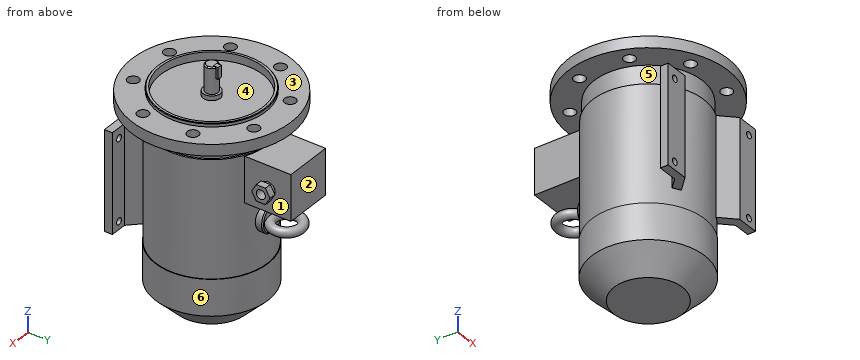
```python
from build123d import *

# Parameters (mm, degrees)
SKETCH_1_R           = 5.5
EXTRUDE_1_DEPTH      = 23
SKETCH_2_W           = 4
SKETCH_2_H           = 4
EXTRUDE_2_DEPTH      = 0.1
EXTRUDE_2_DEPTH_BACK = 10
SKETCH_3_R           = 7.5
EXTRUDE_11_DEPTH     = 4
SKETCH_16_R          = 70
SKETCH_16_R_2        = 47.5
EXTRUDE_13_DEPTH     = 10
SKETCH_17_R          = 47.5
EXTRUDE_14_DEPTH     = 23
SKETCH_18_R          = 5
CUT_EXTRUDE_4_DEPTH  = 28
SKETCH_20_R          = 49
EXTRUDE_15_DEPTH     = 102
SKETCH_21_R          = 49.5
EXTRUDE_16_DEPTH     = 51
CHAMFER_3_SIZE       = 19.5
EXTRUDE_17_DEPTH     = 87
CUT_EXTRUDE_5_REACH  = 128
SKETCH_23_R          = 2.9
SKETCH_24_W          = 42
SKETCH_24_H          = 40
EXTRUDE_18_DEPTH     = 43
SKETCH_25_R          = 12.5
EXTRUDE_19_DEPTH     = 12
CHAMFER_4_SIZE       = 1
SKETCH_27_R          = 4
CHAMFER_5_SIZE       = 1
SKETCH_28_R          = 47.5
SKETCH_28_R_2        = 45
EXTRUDE_20_DEPTH     = 7
CHAMFER_6_SIZE       = 0.5
SKETCH_29_R          = 6
EXTRUDE_21_DEPTH     = 3
EXTRUDE_22_DEPTH     = 6
SKETCH_31_R          = 4
CUT_EXTRUDE_6_DEPTH  = 10


with BuildPart() as part:
    # Sketch 1 → Extrude 1 (new body)
    with BuildSketch(Plane.XY):
        Circle(SKETCH_1_R)
    extrude(amount=EXTRUDE_1_DEPTH)

    # Sketch 2 → Extrude 2 (add, two sides)
    with BuildSketch(Plane.XY.offset(23)) as extrude_2_sk:
        with Locations((0, 5)):
            Rectangle(SKETCH_2_W, SKETCH_2_H)
    extrude(amount=EXTRUDE_2_DEPTH)
    extrude(extrude_2_sk.sketch, amount=-EXTRUDE_2_DEPTH_BACK)

    # Sketch 3 → Extrude 11 (add)
    with BuildSketch(Plane(origin=(0, 0, 0), x_dir=(-1, 0, 0), z_dir=(0, 0, -1))):
        Circle(SKETCH_3_R)
    extrude(amount=EXTRUDE_11_DEPTH)



with BuildPart() as body_2:
    # Sketch 16 → Extrude 13 (new body)
    with BuildSketch(Plane.XY):
        Circle(SKETCH_16_R)
        Circle(SKETCH_16_R_2, mode=Mode.SUBTRACT)
    extrude(amount=-EXTRUDE_13_DEPTH)


with BuildPart() as part_1:
    add(part.part)

    add(body_2.part)  # Extrude 14 merges body 2
    # Sketch 17 → Extrude 14 (add)
    with BuildSketch(Plane(origin=(0, 0, -4), x_dir=(-1, 0, 0), z_dir=(0, 0, -1))):
        with Locations(Location((0, 0, 0), (0, 0, 180))):  # turned: the seam where the file's is
            Circle(SKETCH_17_R)
    extrude(amount=EXTRUDE_14_DEPTH)

    # Sketch 18 → Cut-Extrude 4 (cut, through all)
    with BuildSketch(Plane.XY):
        with Locations((-22.004297361, 53.123073119)):
            Circle(SKETCH_18_R)
        with Locations((22.004297361, 53.123073119)):
            Circle(SKETCH_18_R)
        with Locations((53.123073119, 22.004297361)):
            Circle(SKETCH_18_R)
        with Locations((53.123073119, -22.004297361)):
            Circle(SKETCH_18_R)
        with Locations((22.004297361, -53.123073119)):
            Circle(SKETCH_18_R)
        with Locations((-22.004297361, -53.123073119)):
            Circle(SKETCH_18_R)
        with Locations((-53.123073119, -22.004297361)):
            Circle(SKETCH_18_R)
        with Locations((-53.123073119, 22.004297361)):
            Circle(SKETCH_18_R)
    extrude(amount=-CUT_EXTRUDE_4_DEPTH, mode=Mode.SUBTRACT)

    # Sketch 20 → Extrude 15 (add)
    with BuildSketch(Plane(origin=(0, 0, -27), x_dir=(-1, 0, 0), z_dir=(0, 0, -1))):
        Circle(SKETCH_20_R)
    extrude(amount=EXTRUDE_15_DEPTH)

    # Sketch 21 → Extrude 16 (add)
    with BuildSketch(Plane(origin=(0, 0, -129), x_dir=(-1, 0, 0), z_dir=(0, 0, -1))):
        Circle(SKETCH_21_R)
    extrude(amount=EXTRUDE_16_DEPTH)

    # Chamfer 3
    chamfer_3_edges = [part_1.edges().sort_by_distance(p)[0] for p in [
        (49.5, 0, -180),
    ]]
    chamfer(chamfer_3_edges, length=CHAMFER_3_SIZE)

    # Sketch 22 → Extrude 17 (add)
    with BuildSketch(Plane.XY.offset(-27)):
        with BuildLine():
            Line((-53, -49), (-53, -56))
            Line((-53, -56), (-44.904134404, -56))
            Line((-44.904134404, -56), (-42, -56))
            Line((-42, -56), (-32.646287703, -56))
            Line((-32.646287703, -56), (-20.944471698, -44.298183995))
            ThreePointArc((-20.944471698, -44.298183995), (-24.169591816, -42.624298603), (-27.261801405, -40.716018766))
            Line((-27.261801405, -40.716018766), (-35.54578264, -49))
            Line((-35.54578264, -49), (-53, -49))
        make_face()
        with BuildLine():
            Line((-26.179896787, -39.634114147), (-27.261801405, -40.716018766))
            ThreePointArc((-27.261801405, -40.716018766), (-24.169591816, -42.624298603), (-20.944471698, -44.298183995))
            Line((-20.944471698, -44.298183995), (-19.815619627, -43.169331924))
            ThreePointArc((-19.815619627, -43.169331924), (-23.065587435, -41.52383263), (-26.179896787, -39.634114147))
        make_face()
        with BuildLine():
            Line((-19.29701834, -32.7512357), (-26.179896787, -39.634114147))
            ThreePointArc((-26.179896787, -39.634114147), (-23.065587435, -41.52383263), (-19.815619627, -43.169331924))
            Line((-19.815619627, -43.169331924), (-14.172440123, -37.52615242))
            Line((-14.172440123, -37.52615242), (-19.29701834, -32.7512357))
        make_face()
        with BuildLine():
            ThreePointArc((28.971766908, -39.517549547), (25.460241586, -41.8661689), (21.759468274, -43.903593707))
            Line((21.759468274, -43.903593707), (33.855874567, -56))
            Line((33.855874567, -56), (42, -56))
            Line((42, -56), (43.639075317, -56))
            Line((43.639075317, -56), (53, -56))
            Line((53, -56), (53, -49))
            Line((53, -49), (38.45421736, -49))
            Line((38.45421736, -49), (28.971766908, -39.517549547))
        make_face()
        with BuildLine():
            Line((15.243541187, -37.38766662), (20.638100121, -42.782225554))
            ThreePointArc((20.638100121, -42.782225554), (24.364898956, -40.775013168), (27.89820479, -38.44398743))
            Line((27.89820479, -38.44398743), (25.07325078, -35.61903342))
            Line((25.07325078, -35.61903342), (15.243541187, -37.38766662))
        make_face()
    extrude(amount=-EXTRUDE_17_DEPTH)

    # Sketch 23 → Cut-Extrude 5 (cut, up to next)
    with BuildSketch(Plane.XZ.offset(56), mode=Mode.PRIVATE) as cut_extrude_5_sk1:
        with Locations(Location((45, -36, 0), (0, 0, 270))):  # turned: the seam where the file's is
            Circle(SKETCH_23_R)
    cut_extrude_5_tool1 = extrude(cut_extrude_5_sk1.sketch, amount=-CUT_EXTRUDE_5_REACH, mode=Mode.PRIVATE) & part_1.part
    add(cut_extrude_5_tool1.solids().sort_by_distance((45, -56, -36))[0], mode=Mode.SUBTRACT)
    # Sketch 23 → Cut-Extrude 5 (cut, up to next)
    with BuildSketch(Plane.XZ.offset(56), mode=Mode.PRIVATE) as cut_extrude_5_sk2:
        with Locations(Location((-45, -36, 0), (0, 0, 270))):  # turned: the seam where the file's is
            Circle(SKETCH_23_R)
    cut_extrude_5_tool2 = extrude(cut_extrude_5_sk2.sketch, amount=-CUT_EXTRUDE_5_REACH, mode=Mode.PRIVATE) & part_1.part
    add(cut_extrude_5_tool2.solids().sort_by_distance((-45, -56, -36))[0], mode=Mode.SUBTRACT)
    # Sketch 23 → Cut-Extrude 5 (cut, up to next)
    with BuildSketch(Plane.XZ.offset(56), mode=Mode.PRIVATE) as cut_extrude_5_sk3:
        with Locations(Location((45, -107, 0), (0, 0, 270))):  # turned: the seam where the file's is
            Circle(SKETCH_23_R)
    cut_extrude_5_tool3 = extrude(cut_extrude_5_sk3.sketch, amount=-CUT_EXTRUDE_5_REACH, mode=Mode.PRIVATE) & part_1.part
    add(cut_extrude_5_tool3.solids().sort_by_distance((45, -56, -107))[0], mode=Mode.SUBTRACT)
    # Sketch 23 → Cut-Extrude 5 (cut, up to next)
    with BuildSketch(Plane.XZ.offset(56), mode=Mode.PRIVATE) as cut_extrude_5_sk4:
        with Locations(Location((-45, -107, 0), (0, 0, 270))):  # turned: the seam where the file's is
            Circle(SKETCH_23_R)
    cut_extrude_5_tool4 = extrude(cut_extrude_5_sk4.sketch, amount=-CUT_EXTRUDE_5_REACH, mode=Mode.PRIVATE) & part_1.part
    add(cut_extrude_5_tool4.solids().sort_by_distance((-45, -56, -107))[0], mode=Mode.SUBTRACT)

    # Sketch 24 → Extrude 18 (add)
    with BuildSketch(Plane(origin=(0, 42, 0), x_dir=(-1, 0, 0), z_dir=(0, 1, 0))):
        with Locations((0, -47.88562837)):
            Rectangle(SKETCH_24_W, SKETCH_24_H)
    extrude(amount=EXTRUDE_18_DEPTH)

    # Sketch 25 → Extrude 19 (add)
    with BuildSketch(Plane(origin=(0, 42, 0), x_dir=(-1, 0, 0), z_dir=(0, 1, 0))):
        with Locations(Location((0, -88, 0), (0, 0, 270))):  # turned: the seam where the file's is
            Circle(SKETCH_25_R)
    extrude(amount=EXTRUDE_19_DEPTH)

    # Chamfer 4
    chamfer_4_edges = [part_1.edges().sort_by_distance(p)[0] for p in [
        (0, 54, -75.5),
    ]]
    chamfer(chamfer_4_edges, length=CHAMFER_4_SIZE)

    # Sweep 1: sweep along a path in Sketch 26
    with BuildLine(Plane.XY.offset(-88)) as sweep_1_path:
        CenterArc((0, 66), 12, 0, 360)
    # Sketch 27 → Sweep 1 (sweep)
    with BuildSketch(Plane(origin=(0, 0, 0), x_dir=(0, 0, -1), z_dir=(1, 0, 0))):
        with Locations((88, 78)):
            Circle(SKETCH_27_R)
    sweep(path=sweep_1_path.line)

    # Chamfer 5
    chamfer_5_edges = [part_1.edges().sort_by_distance(p)[0] for p in [
        (-3.102418411, -4.541475531, 23),
    ]]
    chamfer(chamfer_5_edges, length=CHAMFER_5_SIZE)

    # Sketch 28 → Extrude 20 (add)
    with BuildSketch(Plane.XY.offset(-4)):
        Circle(SKETCH_28_R)
        Circle(SKETCH_28_R_2, mode=Mode.SUBTRACT)
    extrude(amount=EXTRUDE_20_DEPTH)

    # Chamfer 6
    chamfer_6_edges = [part_1.edges().sort_by_distance(p)[0] for p in [
        (-47.5, 0, 3),
    ]]
    chamfer(chamfer_6_edges, length=CHAMFER_6_SIZE)

    # Sketch 29 → Extrude 21 (add)
    with BuildSketch(Plane(origin=(21, 0, 0), x_dir=(0, 0, -1), z_dir=(1, 0, 0))):
        with Locations(Location((47.88562837, 65, 0), (0, 0, 180))):  # turned: the seam where the file's is
            Circle(SKETCH_29_R)
    extrude(amount=EXTRUDE_21_DEPTH)

    # Sketch 30 → Extrude 22 (add)
    with BuildSketch(Plane(origin=(24, 0, 0), x_dir=(0, 0, -1), z_dir=(1, 0, 0))):
        Polygon((47.88562837, 73.082903769), (40.88562837, 69.041451884), (40.88562837, 60.958548116), (47.88562837, 56.917096231), (54.88562837, 60.958548116), (54.88562837, 69.041451884), align=None)
    extrude(amount=EXTRUDE_22_DEPTH)

    # Sketch 31 → Cut-Extrude 6 (cut)
    with BuildSketch(Plane(origin=(30, 0, 0), x_dir=(0, 0, -1), z_dir=(1, 0, 0))):
        with Locations((47.88562837, 65)):
            Circle(SKETCH_31_R)
    extrude(amount=-CUT_EXTRUDE_6_DEPTH, mode=Mode.SUBTRACT)


solid = part_1.part
```
Part model, mm, in its own coordinate system. Face numbers are marked on the shaded views. A direction names the side the tool comes from. Coordinates: 2 decimals unless noted, no trailing zeros. Order: outer loops, then holes, each group sorted by start corner. A loop starts at its lowest first (then second) coordinate and runs counter-clockwise, first axis right, second up. Notation, with made-up numbers: (-27.75, 24) - (-7.75, 24) arc R36 ccw to (-7.75, 59) - close; hole circle Ø4 at (-26.75, 1.25). An arc over 180 degrees is marked (long way). Return JSON: item names as keys, results as strings. Group by question number.
Item 1: Which spindle directions (+Z, -Z, +X, -X, +Y, -Y) get a long thin tool onto all of the face, cutting with end or side? Do the marked faces 4, 5 and 6. Say none if no direction does.
Item 2: Cut at B-B (z = -60). List the corners of the cut face in (x, y).
Item 3: Cut at A-A (z = -107). List the corners of the cut face in (x, y).
Item 4: Pull direction Y, two halves, no side cores. Call the marked faces 1, 2 and 3: pulls with the +Y half, pulls with the -Y half, needs draft (parallel to the pull), parting line crosses it, or undercut.
Item 5: Cut at C-C (z = 6.5). List the corners of the cut face in (x, y), plus the area to 3 significant figures.
Item 6: Drill centre lines: probe 1 along Z at (x, y) = (19, -18); probe 2 along X at (y, z) = (-1, -51); probe 3 along Z at (x, y) = (57, 8.5). Where is each one in solid material? Low to high. Write a range as from..to.
Item 7: Pin check, flat tips, straight feed: pin 1 (20 mm diameter, centred on y = 62.5, z = -38.5, fed in from +X); pin 2 (5 mm diameter, centred on x = 26, y = 63.5, fed in from +Z); pin 3 (5 mm diameter, centred on x = -46.5, z = -82, fed in from +Y). Stop position of each tip, or through.
Check values:
{
 "1": {"face 4": "+Z", "face 5": "none", "face 6": "-Z"},
 "2": {"outline": "(-53, -56) - (-32.65, -56) - (-20.94, -44.3) arc R49 ccw to (21.76, -43.9) - (33.86, -56) - (53, -56) - (53, -49) - (38.45, -49) - (28.97, -39.52) arc R49 ccw to (21, 44.27) - (21, 85) - (-21, 85) - (-21, 44.27) arc R49 ccw to (-27.26, -40.72) - (-35.55, -49) - (-53, -49) - close"},
 "3": {"outline": "(-53, -56) - (-47.9, -56) - (-47.9, -49) - (-53, -49) - close; (-42.1, -56) - (-32.65, -56) - (-20.94, -44.3) arc R49 ccw to (21.76, -43.9) - (33.86, -56) - (42.1, -56) - (42.1, -49) - (38.45, -49) - (28.97, -39.52) arc R49 ccw (long way) to (-27.26, -40.72) - (-35.55, -49) - (-42.1, -49) - close; (47.9, -56) - (53, -56) - (53, -49) - (47.9, -49) - close"},
 "4": {"face 1": "undercut", "face 2": "pulls with the +Y half", "face 3": "needs draft"},
 "5": {"outline": "circle Ø11 at (0, 0)", "area": "95.0 mm2"},
 "6": {"probe 1": "z = -180..-4", "probe 2": "x = -48.99..48.99", "probe 3": "z = -10..0"},
 "7": {"pin 1": "stops at x = 30", "pin 2": "stops at z = 0", "pin 3": "stops at y = 21.56"}
}
